The model under review builds one solid part; all positions refer to its coordinate system, in mm. Round coordinates to 2 decimals unless told otherwise and drop trailing zeros. Write each loop counter-clockwise with the first axis right and the second up, starting at its lowest first coordinate (ties: lowest second). Pieces come first, ordered by that corner, then holes. Notation, with made-up numbers: (47, 0) -> (70, 0) arc R20 cw to (70, 27) -> close; hole circle Ø11 at (42.25, 33.5). An arc over 180 degrees is marked (long way). Use CSV: the item, a comma, the result in double quotes. Start each with the question number.
1) Take a section at C-C, the plane z = 42. Give the boundary of the cut face in (x, y), then the cut area to 3 significant figures.
2) Wall thickness on probe 1 along X at (y, z) = (0.5, 104); probe 2 along Z at (x, y) = (-3, 6.25); probe 3 along X at (y, z) = (-11, 255): over which ranges is each line inside the solid? List them lowest first. Write a range as [from, to].
3) Take a section at A-A, the plane x = 0. Give the boundary of the cut face in (y, z), then the cut area to 3 significant figures.
4) For pin 1 Ø12 at (x, z) = (-9.5, 254) entering from +Y; pin 2 Ø4 at (x, z) = (-8.5, 284.5) entering from +Y; pin 3 Ø3 at (x, z) = (7.5, 252.5) entering from +Y, all flat-tipped, find the tip position at first contact; note any pin that passes through.
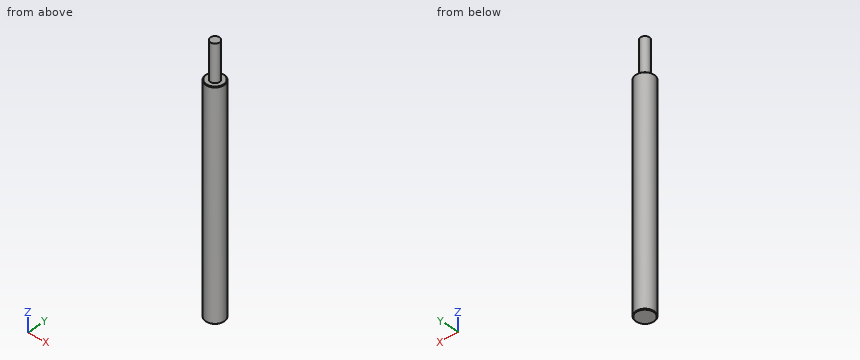
from build123d import *

# Parameters (mm, degrees)
F0_R     = 12.7
F1_DEPTH = 304.8
F2_SIZE  = 0.762
F3_R     = 6.35
F4_DEPTH = 50.8


with BuildPart() as f1:
    # F0 (on Top) → F1 (new body)
    with BuildSketch(Plane.XY):
        Circle(F0_R)
    extrude(amount=F1_DEPTH)

    # F2
    f2_edges = [f1.edges().sort_by_distance(p)[0] for p in [
        (-12.7, 0, 0),
        (-12.7, 0, 304.8),
    ]]
    chamfer(f2_edges, length=F2_SIZE)

    # F3 (on face) → F4 (join)
    with BuildSketch(Plane.XY.offset(304.8)):
        Circle(F3_R)
    extrude(amount=F4_DEPTH)


solid = f1.part
Values found:
1,outline,"circle Ø25.4 at (0, 0)"
1,area,"507 mm²"
2,probe 1,"[-12.69, 12.69]"
2,probe 2,"[0, 304.8]"
2,probe 3,"[-6.35, 6.35]"
3,outline,"(-12.7, 0.76) -> (-11.94, 0) -> (11.94, 0) -> (12.7, 0.76) -> (12.7, 304.04) -> (11.94, 304.8) -> (6.35, 304.8) -> (6.35, 355.6) -> (-6.35, 355.6) -> (-6.35, 304.8) -> (-11.94, 304.8) -> (-12.7, 304.04) -> close"
3,area,"8,390 mm²"
4,pin 1,"y = 12.21"
4,pin 2,"y = 10.91"
4,pin 3,"y = 11.19"
